Here's how the part is built. I have some questions about the finished solid (model axes, mm). Face numbers are marked on the shaded views. A direction names the side the tool comes from. Give positions to 0.01 mm unless a question says otherwise; leave off trailing zeros. Order: outer loops, then holes, each group sorted by start corner. A loop starts at its lowest first (then second) coordinate and runs counter-clockwise, first axis right, second up. Notation, with made-up numbers: M -39.75,70 L 2.25,70 A14 ccw 2.25,94 Z; hole C 73,-8.75 d4. An arc over 180 degrees is marked long. Use CSV: the item, a comma, the result in double quotes. Start each with the question number.
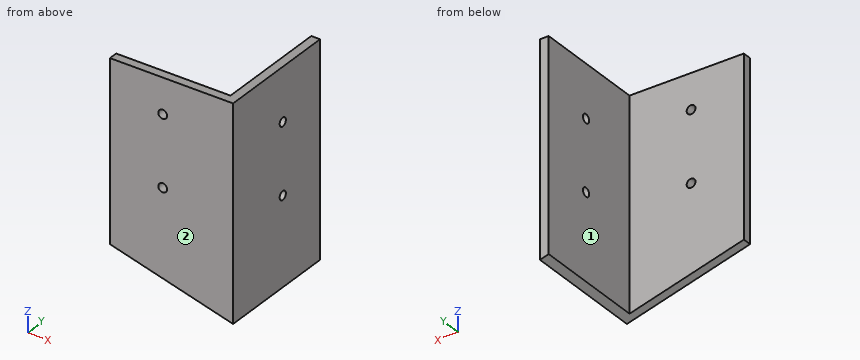
Autodesk Inventor part; units mm, degrees
ref_plane "Work Plane1" through (0, 0, 0) normal (-0.2588, 0, -0.9659) x (0, 1, 0)
ref_plane "YZ Plane" through (0, 0, 0) normal (1, 0, 0) x (0, 1, 0)
ref_plane "XZ Plane" through (0, 0, 0) normal (0, 1, 0) x (-1, 0, 0)
sketch "Sketch1" plane through (0, 0, 0) normal (0, 0, 1) x (1, 0, 0)
  line L0 (0, 0) -> (0, 44.45)
  line L1 (0, 0) -> (-44.45, 0)
  line L2 (-3.175, 44.45) -> (-3.175, 3.175)
  line L3 (-3.175, 3.175) -> (-44.45, 3.175)
  line L4 (-3.175, 44.45) -> (0, 44.45)
  line L5 (-44.45, 3.175) -> (-44.45, 0)
  dimension "d0" = 44.45
  dimension "d1" = 44.45
  dimension "d2" = 3.175
extrude "Extrusion1" add sketch "Sketch1" along normal blind 76.2
ref_plane "Work Plane1" through (0, 0, 0) normal (-0.2588, 0, -0.9659) x (0, 1, 0)
split "Split1" plane through (0, 0, 0) removes the side toward (-0.2588, 0, -0.9659)
sketch "Sketch2" plane through (-44.45, 3.175, 76.2) normal (0, 1, 0) x (1, 0, 0)
  line L0 (0, 0) -> (44.45, 0)
  circle A0 centre (19.05, 12.7) radius 2.0125
  circle A1 centre (19.05, 38.1) radius 1.8125
  line L1 (0, 64.2897) -> (0, 0)
  point P0 (44.45, 76.2)
  dimension "d6" = 12.7
  dimension "d7" = 25.4
  dimension "d28" = 19.05
  dimension "d29" = 19.05
hole "Hole1" at (-25.4, 3.175, 38.1) at (-25.4, 3.175, 63.5) direction (0, -1, 0) diameter 3.175 end through all
sketch "Sketch3" plane through (-3.175, 3.175, 76.2) normal (-1, 0, 0) x (0, 0, 1)
  line L0 (0, -3.175) -> (0, 41.275)
  line L1 (-75.3493, 41.275) -> (-75.3493, 0)
  circle A0 centre (-19.05, 22.225) radius 1.7587
  circle A1 centre (-44.45, 22.225) radius 1.632
  line L2 (-75.3493, 41.275) -> (0, 41.275)
  point P0 (-76.2, -3.175)
  dimension "d15" = 19.05
  dimension "d16" = 25.4
  dimension "d26" = 19.05
  dimension "d27" = 19.05
hole "Hole2" at (-3.175, 25.4, 31.75) at (-3.175, 25.4, 57.15) direction (1, 0, 0) diameter 3.175 end through all
properties part number "ring support right" material "Aluminum 6061"
Q1. I need wall thicknesses on line 1 (Z direction, x = -25, y = 1); line 2 (Z direction, x = -25.4, y = 2.45); line 3 (Y direction, x = -2.25, z = 31.75). Which ranges of each line are inside material? Lowest first, please. Write a range as [from, to].
Q2. For P1, Ø3, axis at x = -38, z = 12, coming from the +Y side (3 decimals); P2, Ø5, axis at y = 25.4, z = 57.15, coming from the -X side (3 decimals), each with a flat end and sliding along its axis, tell me the tip position at first contact or that it passes through.
Q3. Imagine slicing it at D-D, the plane y = 32. Please give me the cut outline in (x, z) (3 decimals), then the cut area to 3 significant figures.
Q4. Imagine slicing it at C-C, the plane z = 16. Please give me the cut outline in (x, y) (3 decimals), then the cut area to 3 significant figures.
Q5. For the marked faces 1 and 2, which set-ups out of +Z, -Z, +X, -X, +Y, -Y let a thin tool reach every point of the face, with its end or its side?
Q6. Imagine slicing it at B-B, the plane x = -25.4. Please give me the cut outline in (y, z) (1 decimal), then the cut area to 3 significant figures.
Reply:
1,line 1,"z = [6.7, 36.56], [39.64, 61.96], [65.04, 76.2]"
1,line 2,"z = [6.81, 36.51], [39.69, 61.91], [65.09, 76.2]"
1,line 3,"y = [0, 23.81], [26.99, 44.45]"
2,P1,"stops at y = 3.175"
2,P2,"stops at x = -3.175"
3,outline,"M -3.175,0.851 L 0,0 L 0,76.2 L -3.175,76.2 Z"
3,area,"241 mm^2"
4,outline,"M -44.45,0 L 0,0 L 0,44.45 L -3.175,44.45 L -3.175,3.175 L -44.45,3.175 Z"
4,area,"272 mm^2"
5,face 1,"+Z, -Z, -X, +Y"
5,face 2,"+Z, -Z, +X, -X, -Y"
6,outline,"M 0,6.8 L 3.2,6.8 L 3.2,36.5 L 0,36.5 Z; M 0,39.7 L 3.2,39.7 L 3.2,61.9 L 0,61.9 Z; M 0,65.1 L 3.2,65.1 L 3.2,76.2 L 0,76.2 Z"
6,area,"200 mm^2"
